```python
from build123d import *

# Parameters (mm, degrees)
SKETCH1_W           = 100
SKETCH1_H           = 100
BOSS_EXTRUDE1_DEPTH = 100
SKETCH3_R           = 15
CUT_EXTRUDE1_DEPTH  = 10
SKETCH5_R           = 10
CUT_EXTRUDE2_DEPTH  = 10
SKETCH8_R           = 13
CUT_EXTRUDE3_DEPTH  = 10
SKETCH12_R          = 12.5
CUT_EXTRUDE4_DEPTH  = 10
CUT_EXTRUDE5_START  = -10
SKETCH13_R          = 10
CUT_EXTRUDE5_DEPTH  = 10
SKETCH14_R          = 10
CUT_EXTRUDE6_DEPTH  = 10
FILLET6_R           = 5


with BuildPart() as part:
    # Sketch1 → Boss-Extrude1 (new body)
    with BuildSketch(Plane(origin=(0, 0, 0), x_dir=(1, 0, 0), z_dir=(0, 1, 0))):
        Rectangle(SKETCH1_W, SKETCH1_H)
    extrude(amount=BOSS_EXTRUDE1_DEPTH)

    # Sketch3 → Cut-Extrude1 (cut)
    with BuildSketch(Plane(origin=(0, 100, 0), x_dir=(1, 0, 0), z_dir=(0, 1, 0))):
        with Locations(Location((0, 0, 0), (0, 0, 270))):
            Circle(SKETCH3_R)
    extrude(amount=-CUT_EXTRUDE1_DEPTH, mode=Mode.SUBTRACT)

    # Sketch5 → Cut-Extrude2 (cut)
    with BuildSketch(Plane.XY.offset(50)):
        with Locations((0, 50)):
            Circle(SKETCH5_R)
        with Locations((24.748737342, 74.748737342)):
            Circle(SKETCH5_R)
        with Locations((-24.748737342, 25.251262658)):
            Circle(SKETCH5_R)
    extrude(amount=-CUT_EXTRUDE2_DEPTH, mode=Mode.SUBTRACT)

    # Sketch8 → Cut-Extrude3 (cut)
    with BuildSketch(Plane.ZY.offset(50)):
        with Locations((-16.970562748, 66.970562748)):
            Circle(SKETCH8_R)
        with Locations((16.970562748, 33.029437252)):
            Circle(SKETCH8_R)
    extrude(amount=-CUT_EXTRUDE3_DEPTH, mode=Mode.SUBTRACT)

    # Sketch12 → Cut-Extrude4 (cut)
    with BuildSketch(Plane(origin=(50, 0, 0), x_dir=(0, 0, -1), z_dir=(1, 0, 0))):
        with Locations((-25, 75)):
            Circle(SKETCH12_R)
        with Locations((25, 75)):
            Circle(SKETCH12_R)
        with Locations((25, 25)):
            Circle(SKETCH12_R)
        with Locations((-25, 25)):
            Circle(SKETCH12_R)
    extrude(amount=-CUT_EXTRUDE4_DEPTH, mode=Mode.SUBTRACT)

    # Sketch13 → Cut-Extrude5 (cut)
    with BuildSketch(Plane(origin=(0, 0, -50), x_dir=(-1, 0, 0), z_dir=(0, 0, -1)).offset(CUT_EXTRUDE5_START)):
        with Locations(Location((0, 50, 0), (0, 0, 180))):
            Circle(SKETCH13_R)
        with Locations((-27.5, 77.5)):
            Circle(SKETCH13_R)
        with Locations((27.5, 77.5)):
            Circle(SKETCH13_R)
        with Locations((27.5, 22.5)):
            Circle(SKETCH13_R)
        with Locations((-27.5, 22.5)):
            Circle(SKETCH13_R)
    extrude(amount=CUT_EXTRUDE5_DEPTH, mode=Mode.SUBTRACT)

    # Sketch14 → Cut-Extrude6 (cut)
    with BuildSketch(Plane(origin=(0, 0, 0), x_dir=(-1, 0, 0), z_dir=(0, -1, 0))):
        with Locations(Location((-16.67, 0, 0), (0, 0, 90))):
            Circle(SKETCH14_R)
        with Locations(Location((16.67, 0, 0), (0, 0, 90))):
            Circle(SKETCH14_R)
        with Locations(Location((16.67, 25, 0), (0, 0, 90))):
            Circle(SKETCH14_R)
        with Locations(Location((-16.67, 25, 0), (0, 0, 90))):
            Circle(SKETCH14_R)
        with Locations(Location((-16.67, -25, 0), (0, 0, 90))):
            Circle(SKETCH14_R)
        with Locations(Location((16.67, -25, 0), (0, 0, 90))):
            Circle(SKETCH14_R)
    extrude(amount=-CUT_EXTRUDE6_DEPTH, mode=Mode.SUBTRACT)

    # Fillet6
    fillet6_edges = [part.edges().sort_by_distance(p)[0] for p in [
        (0, 100, -50),
        (50, 100, 0),
        (0, 100, 50),
        (50, 0, 0),
        (0, 0, -50),
        (-50, 0, 0),
        (0, 0, 50),
        (-50, 100, 0),
        (50, 50, 50),
        (50, 50, -50),
        (-50, 50, -50),
        (-50, 50, 50),
    ]]
    fillet(fillet6_edges, radius=FILLET6_R)


solid = part.part
```
Verification items for the finished model (mm, model axes). A direction names the side the tool comes from. Coordinates: 2 decimals unless noted, no trailing zeros. Write each loop counter-clockwise with the first axis right and the second up, starting at its lowest first coordinate (ties: lowest second). Pieces come first, ordered by that corner, then holes. Notation, with made-up numbers: (84, 77.5) - (109, 77.5) arc R27 ccw to (109, 108.5) - close; hole circle Ø9 at (41.5, 6). An arc over 180 degrees is marked (long way). One line per question, with ' | ' between items. Start each with the question number.
1. Draft check along Y on faces 1 (the cylindrical face through (-49, 51, 48)), 2 (the flat face through (0, 50, -40)), 3 (the cylindrical face through (1, 1, -48)), 4 (the cylindrical face through (-37.04, 25.5, -44.93)). Enter one of: released by +Y, released by -Y, zero draft, split by the parting line, or undercut.
2. Section check B-B (y = 50). Enter the section's corners in (x, z), plus the area to 3 significant figures.
3. Section check A-A (x = 0). Enter the section's corners in (y, z), plus the area to 3 significant figures.
4. Material ranges on line 1 along X through (y, z) = (6.5, 0); line 2 along Y through (x, z) = (0, -45.25); line 3 along Y through (x, z) = (44, 25), recorded low to high.
5. Access from +Z, -Z, +X, -X, +Y, -Y to the whole of each face (thin tool, end or side, straight path). Record for faces 5 (the cylindrical face through (-45.07, 79.86, -18.66)), 6 (the flat face through (-27, 23, -40)), 7 (the flat face through (40, 75, -25)).
6. Gauge pin test, flat ends, axial feed: P1, Ø1, axis at y = 31.5, z = 9.5, coming from the -X side; P2, Ø1.5, axis at x = -24, y = 14.5, coming from the -Z side; P3, Ø18, axis at x = -16.67, z = 0, coming from the -Y side. Record the tip position at first contact, or that the pin passes through.
7. Section check C-C (x = -43.5). Enter the section's corners in (y, z).
8. Section check D-D (z = 8). Enter the section's corners in (x, y).
Computed values:
1) face 1: zero draft | face 2: undercut | face 3: released by -Y | face 4: undercut
2) outline: (-50, -45) arc R5 ccw to (-45, -50) - (-10, -50) - (-10, -40) - (10, -40) - (10, -50) - (45, -50) arc R5 ccw to (50, -45) - (50, 45) arc R5 ccw to (45, 50) - (10, 50) - (10, 40) - (-10, 40) - (-10, 50) - (-45, 50) arc R5 ccw to (-50, 45) - close | area: 9,580 mm²
3) outline: (0, -45) arc R5 ccw to (5, -50) - (40, -50) - (40, -40) - (60, -40) - (60, -50) - (95, -50) arc R5 ccw to (100, -45) - (100, -15) - (90, -15) - (90, 15) - (100, 15) - (100, 45) arc R5 ccw to (95, 50) - (60, 50) - (60, 40) - (40, 40) - (40, 50) - (5, 50) arc R5 ccw to (0, 45) - close | area: 9,280 mm²
4) line 1: -50 to -26.67, -6.67 to 6.67, 26.67 to 50 | line 2: 0.01 to 40, 60 to 99.99 | line 3: 0 to 12.5, 37.5 to 62.5, 87.5 to 100
5) face 5: -X | face 6: -Z | face 7: +X
6) P1: x = -40 | P2: z = -40 | P3: y = 10
7) outline: (0, -45) arc R5 ccw to (5, -50) - (95, -50) arc R5 ccw to (100, -45) - (100, 45) arc R5 ccw to (95, 50) - (5, 50) arc R5 ccw to (0, 45) - close; hole circle Ø26 at (33.03, 16.97); hole circle Ø26 at (66.97, -16.97)
8) outline: (-50, 5) arc R5 ccw to (-45, 0) - (-22.67, 0) - (-22.67, 10) - (-10.67, 10) - (-10.67, 0) - (10.67, 0) - (10.67, 10) - (22.67, 10) - (22.67, 0) - (45, 0) arc R5 ccw to (50, 5) - (50, 95) arc R5 ccw to (45, 100) - (12.69, 100) - (12.69, 90) - (-12.69, 90) - (-12.69, 100) - (-45, 100) arc R5 ccw to (-50, 95) - (-50, 42.44) - (-40, 42.44) - (-40, 23.62) - (-50, 23.62) - close
